The figure shows three views and two pictorial views of one solid part (mm, origin at its lowest corner). Answer the questions. A direction names the side the tool comes from. Round coordinates to 2 decimals unless told otherwise and drop trailing zeros. Order: outer loops, then holes, each group sorted by start corner. A loop starts at its lowest first (then second) coordinate and runs counter-clockwise, first axis right, second up. Notation, with made-up numbers: M -35,83.25 L -15,83.25 A32 cw -15,110.25 Z; hole C 10.5,17.5 d10. An arc over 180 degrees is marked long. Return JSON: item names as keys, results as strings.
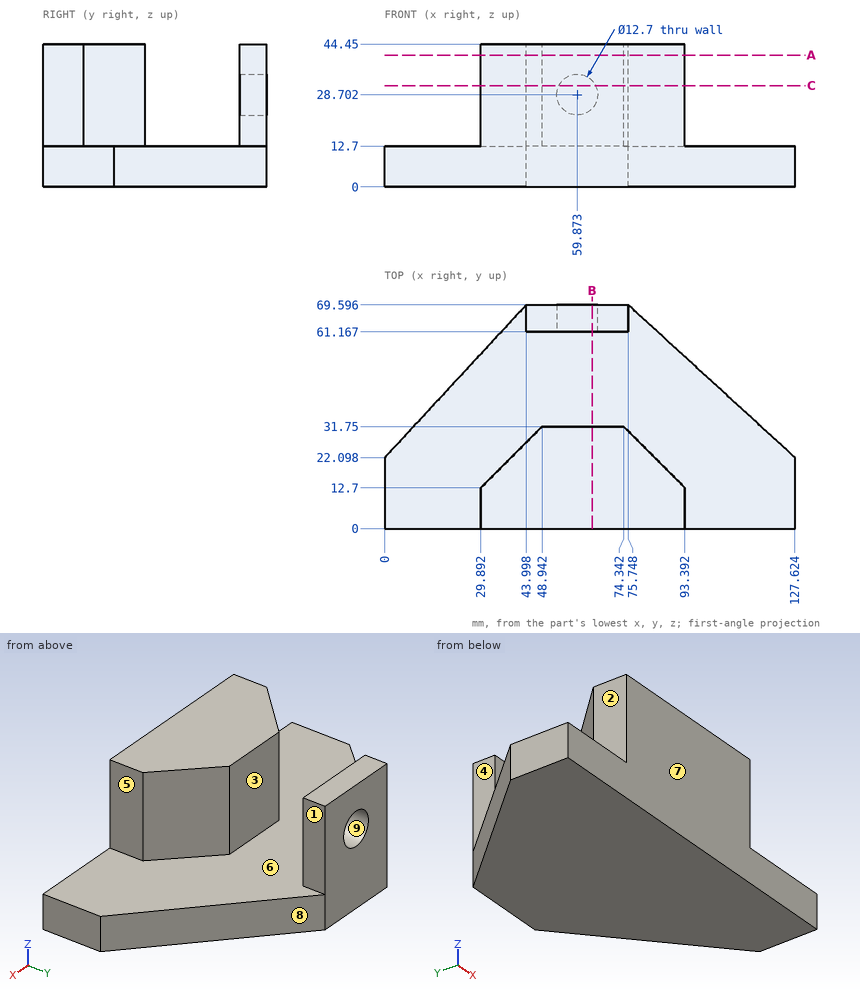
Item 1: Find section A-A (z = 41). Determine the outline of the cut face in (x, y).
Output:
{"outline": "M 29.89,0 L 93.39,0 L 93.39,12.7 L 74.34,31.75 L 48.94,31.75 L 29.89,12.7 Z; M 44,61.17 L 75.75,61.17 L 75.75,69.6 L 44,69.6 Z"}
Item 2: Find section B-B (x = 64.5). Determine the outline of the cut face in (y, z).
Output:
{"outline": "M 0,0 L 69.6,0 L 69.6,24.35 L 61.17,24.35 L 61.17,12.7 L 31.75,12.7 L 31.75,44.45 L 0,44.45 Z; M 61.17,33.05 L 69.6,33.05 L 69.6,44.45 L 61.17,44.45 Z"}
Item 3: Find section C-C (z = 31.5). Determine the outline of the cut face in (x, y), plus the area to 3 significant figures.
Output:
{"outline": "M 29.89,0 L 93.39,0 L 93.39,12.7 L 74.34,31.75 L 48.94,31.75 L 29.89,12.7 Z; M 44,61.17 L 54.17,61.17 L 54.17,69.6 L 44,69.6 Z; M 65.57,61.17 L 75.75,61.17 L 75.75,69.6 L 65.57,69.6 Z", "area": "1,820 mm^2"}
Item 4: The mould has two halves that part along Y. Classify the marked faces 6, 7, 8 and 9: pulls with the +Y half, pulls with the -Y half, needs draft (parallel to the pull), parting line crosses it, or undercut.
Output:
{"face 6": "undercut", "face 7": "pulls with the -Y half", "face 8": "pulls with the +Y half", "face 9": "needs draft"}
Item 5: Which of the six approach directions +Z, -Z, +X, -X, +Y, -Y give full straight-line access (tool end or side, diameter ignored) to the marked faces 1, 2, 3, 4 and 5?
Output:
{"face 1": "+Z, +X, +Y", "face 2": "+Z, -X, +Y, -Y", "face 3": "+Z, +X, -X", "face 4": "+Z, -X, +Y", "face 5": "+Z, +X, +Y, -Y"}
Item 6: Consider line 1 along Y through (x, z) = (68.5, 32); line 2 along X through (y, z) = (12, 40.5); line 3 along Z through (x, y) = (91, 40). Determine where each line is inside the solid, lowest interval first. Write a range as [from, to].
Output:
{"line 1": "y = [0, 31.75], [61.17, 69.6]", "line 2": "x = [29.89, 93.39]", "line 3": "z = [0, 12.7]"}
Item 7: Each of these flat-tipped pins is pushed along its axis until it touches: pin 1 (4 mm diameter, centred on y = 67.5, z = 27, fed in from -X); pin 2 (4 mm diameter, centred on y = 3.5, z = 28.5, fed in from +X); pin 3 (14 mm diameter, centred on y = 4, z = 28, fed in from -X). Where does it stop, or does it pass through?
Output:
{"pin 1": "stops at x = 44", "pin 2": "stops at x = 93.39", "pin 3": "stops at x = 29.89"}
